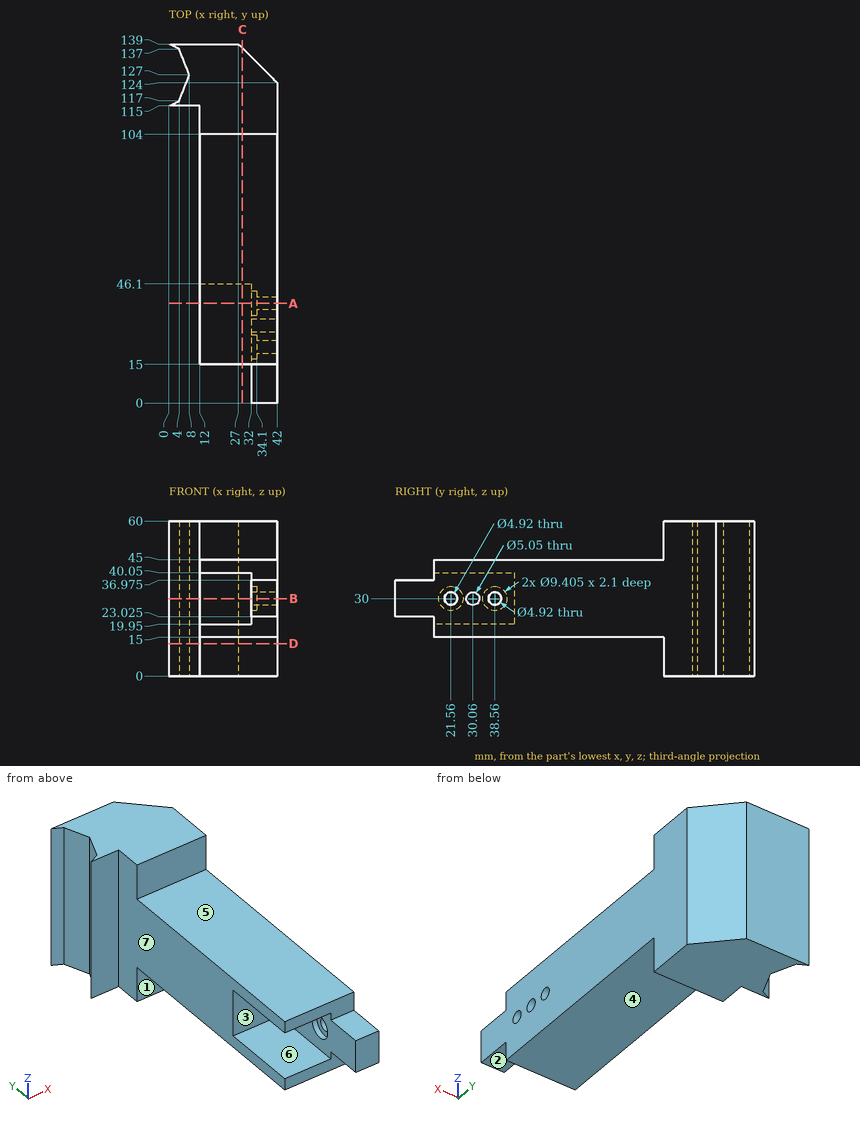
Geometry check sheet. Reference: drawing and pictorial views, mm from the part's lowest x, y, z. A direction names the side the tool comes from. Round coordinates to 2 decimals unless told otherwise and drop trailing zeros. Order: outer loops, then holes, each group sorted by start corner. A loop starts at its lowest first (then second) coordinate and runs counter-clockwise, first axis right, second up.
Q1. Cross-section at C-C, the plane x = 28.5. Enter the section's corners in (y, z), plus the area to 3 significant figures.
Filled sheet:
outline: (15, 15) - (104, 15) - (104, 0) - (137.5, 0) - (137.5, 60) - (104, 60) - (104, 45) - (15, 45) - (15, 40.05) - (46.1, 40.05) - (46.1, 19.95) - (15, 19.95) - close
area: 4,050 mm2
Q2. Cross-section at A-A, the plane y = 38.56. Enter the section's corners in (x, z).
Filled sheet:
outline: (12, 15) - (42, 15) - (42, 27.54) - (34.1, 27.54) - (34.1, 25.3) - (32, 25.3) - (32, 19.95) - (12, 19.95) - close; (12, 40.05) - (32, 40.05) - (32, 34.7) - (34.1, 34.7) - (34.1, 32.46) - (42, 32.46) - (42, 45) - (12, 45) - close
Q3. Scan lines: L1, parallel to Z at x = 28, y = 35; L2, parallel to Y at x = 35.5, z = 30 (3 decimals); L3, parallel to X at y = 75.5, z = 39.5. Record each from-to range of solid material in increasing order.
Filled sheet:
L1: z = 15 to 19.95, 40.05 to 45
L2: y = 0 to 19.1, 24.02 to 27.535, 32.585 to 36.1, 41.02 to 130.5
L3: x = 12 to 42
Q4. Cross-section at B-B, the plane z = 30. Give the number of separate pieces and of enclosed holes in the cut face, plus the area to 3 significant figures.
Filled sheet:
separate pieces: 4
enclosed holes: 0
area: 3,130 mm2
Q5. Set-up check for the marked faces 4, 5, 6 and 7: record each of +Z, -Z, +X, -X, +Y, -Y from which the full face is reachable in a straight line by a thin tool's end or side.
Filled sheet:
face 4: -Z, +X, -X, -Y
face 5: +Z, +X, -X, -Y
face 6: -X, -Y
face 7: +Z, -Z, -X, -Y
Q6. Draft check along Z on the marked faces 1, 2 and 3. Enter one of: pulls with the +Z half, pulls with the -Z half, needs draft (parallel to the pull), parting line crosses it, or undercut.
Filled sheet:
face 1: needs draft
face 2: pulls with the -Z half
face 3: undercut
Q7. Cross-section at D-D, the plane z = 12.5. Enter the section's corners in (x, y), plus the area to 3 significant figures.
Filled sheet:
outline: (0, 115) - (12, 115) - (12, 104) - (42, 104) - (42, 124) - (27, 139) - (0, 139) - (4, 137) - (8, 127) - (4, 117) - close
area: 1,100 mm2
Q8. Depth check by flat-ended pin: P1, Ø4.5, axis at y = 20, z = 30, coming from the -X side; P2, Ø5, axis at x = 5.5, z = 48.5, coming from the -Y side; P3, Ø4.5, axis at x = 20.5, z = 49.5, coming from the -Y side. Enter the tip coordinate at first touch or a pass-through.
Filled sheet:
P1: stops at x = 34.1
P2: stops at y = 115
P3: stops at y = 104
